from build123d import *

# Parameters (mm, degrees)
SKETCH_R        = 31.501905
PAD_DEPTH       = 100
SKETCH001_W     = 8.851912
SKETCH001_H     = 63.773734
POCKET_DEPTH    = 8.5
POCKET001_DEPTH = 7.5


with BuildPart() as part:
    # Sketch (on Sketch) → Pad (new body)
    with BuildSketch(Plane.XY):
        Circle(SKETCH_R)
    extrude(amount=PAD_DEPTH)

    # Sketch001 (on Sketch) → Pocket (cut, symmetric)
    with BuildSketch(Plane(origin=(-2, -31, 0), x_dir=(1, 0, 0), z_dir=(0, -1, 0))):
        with Locations((2.276907, 41.234547)):
            Rectangle(SKETCH001_W, SKETCH001_H)
    extrude(amount=POCKET_DEPTH, both=True, mode=Mode.SUBTRACT)

    # Sketch002 → Pocket001 (cut, symmetric)
    with BuildSketch(Plane.YZ.offset(31)):
        with BuildLine():
            ThreePointArc((10.983905, 74.589867), (0, 85.573772), (-10.983905, 74.589867))
            Line((-10.983905, 74.589867), (-10.983905, 30.654249))
            ThreePointArc((-10.983905, 30.654249), (0, 19.670344), (10.983905, 30.654249))
            Line((10.983905, 30.654249), (10.983905, 74.589867))
        make_face()
    extrude(amount=POCKET001_DEPTH, both=True, mode=Mode.SUBTRACT)


solid = part.part
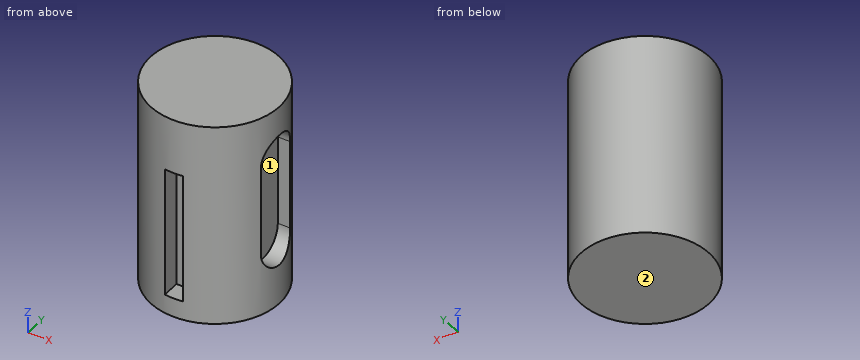
Check sheet for the modelled part. Datum: model origin and axes. Units: mm. Face numbers are marked on the shaded views. A direction names the side the tool comes from. Round coordinates to 2 decimals unless told otherwise and drop trailing zeros. Loops run counter-clockwise (first coordinate to the right, second up) from the corner with the lowest first, then second, coordinate; pieces in that order, holes last. Notation, with made-up numbers: (10, -27.75) - (26, -27.75) arc R10 cw to (26, -12.75) - close; hole circle Ø9 at (64.5, 63.5). An arc over 180 degrees is marked (long way). Answer as CSV lines item,"result". Start each with the question number.
Item 1: Scan lines: line 1 (X direction, y = -23, z = 44); line 2 (Y direction, x = 0, z = 28.5); line 3 (X direction, y = -28, z = 21). Record each from-to range of solid material in increasing order. Write a range as [from, to].
Item 2: Section check D-D (x = 0). Record the boundary of the cut face in (y, z), and give its area (3 significant figures).
Item 3: Section check C-C (y = -24). Record the boundary of the cut face in (x, z), and give its area (3 significant figures).
Item 4: Section check B-B (z = 71.5). Record the boundary of the cut face in (x, y).
Item 5: Depth check by flat-ended pin: P1, Ø5, axis at x = -10.5, z = 41, coming from the +Y side; P2, Ø2.5, axis at x = 1.5, z = 56.5, coming from the -Y side; P3, Ø7, axis at y = -27.5, z = 38, coming from the +X side; P4, Ø1, axis at x = 13.5, y = 10, coming from the -Z side. Enter the tip coordinate at first touch or a pass-through.
Item 6: Set-up check for the marked faces 1 and 2: record each of +Z, -Z, +X, -X, +Y, -Y from which the full face is reachable in a straight line by a thin tool's end or side.
Item 7: Section check A-A (x = 28). Record the boundary of the cut face in (y, z), and give its area (3 significant figures).
Report:
1,line 1,"x = [-21.53, -4.15], [4.7, 21.53]"
1,line 2,"y = [-22.5, 31.5]"
1,line 3,"x = [-14.44, -4.15], [4.7, 14.44]"
2,outline,"(-31.5, 0) - (31.5, 0) - (31.5, 100) - (-31.5, 100) - (-31.5, 73.12) - (-22.5, 73.12) - (-22.5, 9.35) - (-31.5, 9.35) - close"
2,area,"5,730 mm2"
3,outline,"(-20.41, 0) - (20.41, 0) - (20.41, 100) - (-20.41, 100) - close; hole (-4.15, 9.35) - (4.7, 9.35) - (4.7, 73.12) - (-4.15, 73.12) - close"
3,area,"3,520 mm2"
4,outline,"(-4.15, -31.23) - (-4.15, -22.5) - (4.7, -22.5) - (4.7, -31.15) arc R31.5 ccw to (29.52, -10.98) - (23.5, -10.98) - (23.5, 10.98) - (29.52, 10.98) arc R31.5 ccw (long way) to start"
5,P1,"stops at y = 30.47"
5,P2,"stops at y = -22.5"
5,P3,"stops at x = 20.41"
5,P4,"stops at z = 0"
6,face 1,"+X"
6,face 2,"-Z, +X, -X, +Y, -Y"
7,outline,"(-14.44, 0) - (14.44, 0) - (14.44, 100) - (-14.44, 100) - close; hole (-10.98, 30.65) arc R10.98 ccw to (10.98, 30.65) - (10.98, 74.59) arc R10.98 ccw to (-10.98, 74.59) - close"
7,area,"1,540 mm2"
